from build123d import *

# Parameters (mm, degrees)
BOSS_EXTRUDE1_DEPTH      = 30
BOSS_EXTRUDE1_DEPTH_BACK = 30
FILLET1_R                = 5
SKETCH2_R                = 15
CUT_EXTRUDE1_DEPTH       = 124
FILLET2_R                = 30


with BuildPart() as part:
    # Sketch1 → Boss-Extrude1 (new, two sides: drawn at the far end of the back side and taken through both)
    with BuildSketch(Plane.XY.offset(-BOSS_EXTRUDE1_DEPTH_BACK)):
        with BuildLine():
            Line((108, 0), (124, 0))
            Line((124, 0), (124, 68))
            ThreePointArc((124, 68), (111.026334039, 76.540961621), (106, 91.237900077))
            Line((106, 91.237900077), (106, 116))
            Line((106, 116), (92, 116))
            ThreePointArc((92, 116), (62, 86), (32, 116))
            Line((32, 116), (18, 116))
            Line((18, 116), (18, 91.237900077))
            ThreePointArc((18, 91.237900077), (12.973665961, 76.540961621), (0, 68))
            Line((0, 68), (0, 0))
            Line((0, 0), (16, 0))
            Line((16, 0), (16, 54))
            Line((16, 54), (108, 54))
            Line((108, 54), (108, 0))
        make_face()
    extrude(amount=BOSS_EXTRUDE1_DEPTH + BOSS_EXTRUDE1_DEPTH_BACK)

    # Fillet1
    fillet1_edges = [part.edges().sort_by_distance(p)[0] for p in [
        (106, 103.618950039, -30),
        (111.026334039, 76.540961621, -30),
        (18, 103.618950039, 30),
        (12.973665961, 76.540961621, 30),
        (12.973665961, 76.540961621, -30),
        (111.026334039, 76.540961621, 30),
        (106, 103.618950039, 30),
        (18, 103.618950039, -30),
    ]]
    fillet(fillet1_edges, radius=FILLET1_R)

    # Sketch2 → Cut-Extrude1 (cut)
    with BuildSketch(Plane(origin=(124, 0, 0), x_dir=(0, 0, -1), z_dir=(1, 0, 0))):
        with Locations((0, 30)):
            Circle(SKETCH2_R)
    extrude(amount=-CUT_EXTRUDE1_DEPTH, mode=Mode.SUBTRACT)

    # Fillet2
    fillet2_edges = [part.edges().sort_by_distance(p)[0] for p in [
        (116, 0, -30),
        (116, 0, 30),
        (8, 0, -30),
        (8, 0, 30),
    ]]
    fillet(fillet2_edges, radius=FILLET2_R - 0.0001)  # a hair under: the kernel refuses the full size


solid = part.part
Build history of the part. All positions in model axes, mm. A direction names the side the tool comes from. Round coordinates to 2 decimals unless told otherwise and drop trailing zeros. Write each loop counter-clockwise with the first axis right and the second up, starting at its lowest first coordinate (ties: lowest second). Pieces come first, ordered by that corner, then holes. Notation, with made-up numbers: (-9, 8) - (24, 8) arc R16 cw to (24, 20) - close; hole circle Ø3 at (-28, 12). An arc over 180 degrees is marked (long way). Use CSV: the item, a comma, the result in double quotes.
(1) Band-saw the part on B-B (z = -8). Write the cut outline in (x, y).
Response:
outline,"(0, 1.09) - (16, 1.09) - (16, 17.31) - (0, 17.31) - close; (0, 42.69) - (16, 42.69) - (16, 54) - (108, 54) - (108, 42.69) - (124, 42.69) - (124, 68) arc R24 cw to (106, 91.24) - (106, 116) - (92, 116) arc R30 cw to (32, 116) - (18, 116) - (18, 91.24) arc R24 cw to (0, 68) - close; (108, 1.09) - (124, 1.09) - (124, 17.31) - (108, 17.31) - close"
(2) Wall check: line 1 (X direction, y = 6, z = 13.5); line 2 (Y direction, x = 5, z = 0); line 3 (Y direction, x = 12.25, z = 0). Give the ranges that are in metal, low to high.
Response:
line 1,"0 to 16, 108 to 124"
line 2,"0 to 15, 45 to 69.91"
line 3,"0 to 15, 45 to 75.65"
(3) Band-saw the part on A-A (y = 25). Write the cut outline in (x, z).
Response:
outline,"(0, -29.58) - (16, -29.58) - (16, -14.14) - (0, -14.14) - close; (0, 14.14) - (16, 14.14) - (16, 29.58) - (0, 29.58) - close; (108, -29.58) - (124, -29.58) - (124, -14.14) - (108, -14.14) - close; (108, 14.14) - (124, 14.14) - (124, 29.58) - (108, 29.58) - close"
(4) Band-saw the part on C-C (x = 62). Write the cut outline in (y, z).
Response:
outline,"(54, -30) - (86, -30) - (86, 30) - (54, 30) - close"
(5) Pin check, flat tips, straight feed: P1, Ø4, axis at x = 109, y = 72, coming from the -Z side; P2, Ø5, axis at x = 70.5, z = 20, coming from the -Y side; P3, Ø4, axis at x = 17.5, y = 104, coming from the -Z side; P4, Ø1.5, axis at x = 14, z = 23.5, coming from the -Y side. Stop position of each tip, or through.
Response:
P1,"z = -30"
P2,"y = 54"
P3,"z = -28.57"
P4,"y = 10.44"
(6) Band-saw the part on D-D (z = -22). Write the cut outline in (x, y).
Response:
outline,"(0, 9.6) - (16, 9.6) - (16, 54) - (108, 54) - (108, 9.6) - (124, 9.6) - (124, 68) arc R24 cw to (106, 91.24) - (106, 116) - (92, 116) arc R30 cw to (32, 116) - (18, 116) - (18, 91.24) arc R24 cw to (0, 68) - close"
(7) 3-axis set-ups, long thin cutter, end or side, ignore diameter. For faces 5 (the cylindrical face through (19, 103, 28)), 6 (the flat face through (106, 103, 0)), 7 (the flat face through (18, 104, 0)), 8 (the flat face through (61, 54, 0)): which of +Z, -Z, +X, -X, +Y, -Y reach the whole face in a straight line?
Response:
face 5,"+Z, -X, +Y"
face 6,"+Z, -Z, +X, +Y"
face 7,"+Z, -Z, -X, +Y"
face 8,"+Z, -Z, -Y"
(8) Mould opens along X. For faces 1 (the cylindrical face through (105, 104, 28)), 2 (the cylindrical face through (62.66, 86.007, -0.42)), 3 (the flat face through (61, 64, 30)), 4 (the cylindrical face through (13.11, 76.72, -0.35)) say: pulls with the +X half, pulls with the -X half, needs draft (parallel to the pull), parting line crosses it, or undercut.
Response:
face 1,"pulls with the +X half"
face 2,"undercut"
face 3,"needs draft"
face 4,"pulls with the -X half"
